```python
from build123d import *

# Parameters (mm, degrees)
F1_DEPTH  = 19.05
F2_R      = 5.08
F3_W      = 76.2
F3_H      = 101.6
F4_DEPTH  = 9.525
F6_DEPTH  = 12.7
F8_DEPTH  = 25.4
F10_DEPTH = 3.175
F12_DEPTH = 6.35
F14_DEPTH = 6.35


with BuildPart() as f1:
    # F0 (on Top) → F1 (new body)
    with BuildSketch(Plane.XY):
        with BuildLine():
            ThreePointArc((41.275, 47.625), (39.4151280605, 52.1151280605), (34.925, 53.975))
            Line((34.925, 53.975), (-34.925, 53.975))
            ThreePointArc((-34.925, 53.975), (-39.4151280605, 52.1151280605), (-41.275, 47.625))
            Line((-41.275, 47.625), (-41.275, -47.625))
            ThreePointArc((-41.275, -47.625), (-39.4151280605, -52.1151280605), (-34.925, -53.975))
            Line((-34.925, -53.975), (34.925, -53.975))
            ThreePointArc((34.925, -53.975), (39.4151280605, -52.1151280605), (41.275, -47.625))
            Line((41.275, -47.625), (41.275, 47.625))
        make_face()
    extrude(amount=F1_DEPTH)

    # F2
    f2_edges = [f1.edges().sort_by_distance(p)[0] for p in [
        (0, -53.975, 0),
    ]]
    fillet(f2_edges, radius=F2_R)

    # F3 (on face) → F4 (cut)
    with BuildSketch(Plane.XY.offset(19.05)):
        Rectangle(F3_W, F3_H)
    extrude(amount=-F4_DEPTH, mode=Mode.SUBTRACT)

    # F5 (on face) → F6 (cut)
    with BuildSketch(Plane.XY.offset(19.05)):
        with BuildLine():
            ThreePointArc((-34.925, 53.975), (-38.1, 53.124261314), (-40.424261314, 50.8))
            Line((-40.424261314, 50.8), (-38.1, 50.8))
            Line((-38.1, 50.8), (38.1, 50.8))
            Line((38.1, 50.8), (40.424261314, 50.8))
            ThreePointArc((40.424261314, 50.8), (38.1, 53.124261314), (34.925, 53.975))
            Line((34.925, 53.975), (-34.925, 53.975))
        make_face()
    extrude(amount=-F6_DEPTH, mode=Mode.SUBTRACT)

    # F7 (on face) → F8 (cut)
    with BuildSketch(Plane(origin=(38.1, 0, 0), x_dir=(0, -1, 0), z_dir=(-1, 0, 0))):
        Polygon((34.925, 15.875), (34.925, 19.05), (-50.8, 19.05), (-50.8, 9.525), (50.8, 9.525), (50.8, 15.875), align=None)
    extrude(amount=-F8_DEPTH, mode=Mode.SUBTRACT)

    # F9 (on face) → F10 (cut)
    with BuildSketch(Plane.YZ.offset(-38.1)):
        Polygon((50.8, 19.05), (-34.925, 19.05), (-34.925, 15.875), (-50.8, 15.875), (-50.8, 9.525), (50.8, 9.525), align=None)
    extrude(amount=-F10_DEPTH, mode=Mode.SUBTRACT)

    # F11 (on face) → F12 (join)
    with BuildSketch(Plane(origin=(0, 0, 15.875), x_dir=(1, 0, 0), z_dir=(0, 0, -1))):
        with BuildLine():
            Line((38.1, 47.625), (41.275, 47.625))
            ThreePointArc((41.275, 47.625), (41.0586289969, 49.2685009364), (40.424261314, 50.8))
            Line((40.424261314, 50.8), (38.1, 50.8))
            Line((38.1, 50.8), (38.1, 47.625))
        make_face()
    extrude(amount=F12_DEPTH)

    # F13 (on face) → F14 (join)
    with BuildSketch(Plane(origin=(0, 0, 15.875), x_dir=(1, 0, 0), z_dir=(0, 0, -1))):
        with BuildLine():
            ThreePointArc((-40.424261314, 50.8), (-41.0586289969, 49.2685009364), (-41.275, 47.625))
            Line((-41.275, 47.625), (-38.1, 47.625))
            Line((-38.1, 47.625), (-38.1, 50.8))
            Line((-38.1, 50.8), (-40.424261314, 50.8))
        make_face()
    extrude(amount=F14_DEPTH)


solid = f1.part
```
The listing builds one solid part. Answer for the finished solid, in the listing's coordinates (mm). A direction names the side the tool comes from. Give positions to 0.01 mm unless a question says otherwise; leave off trailing zeros. Order: outer loops, then holes, each group sorted by start corner. A loop starts at its lowest first (then second) coordinate and runs counter-clockwise, first axis right, second up.
Item 1: For a pull along Z with two mould halves and no side action, classify faces 4 (the face through (-41.275, 1, 7)), 5 (the face through (39.8, 0.7, 1.5)), 6 (the face through (40, -47.625, 13)) as pulls with the +Z half, pulls with the -Z half, needs draft (parallel to the pull), parting line crosses it, or undercut.
From the geometry:
face 4: needs draft
face 5: pulls with the -Z half
face 6: undercut
Item 2: Find the intervals of material crossed by probe 1 along Y at (x, z) = (-15, 18) (3 decimals); probe 2 along Z at (x, y) = (-21, -43.5) (3 decimals); probe 3 along Y at (x, z) = (28.5, 9) (3 decimals), in increasing order.
From the geometry:
probe 1: y = -53.975 to -50.8
probe 2: z = 0 to 9.525
probe 3: y = -53.975 to 50.8
Item 3: The part is cut by section D-D, the plane y = 43.5. Give the vertices of the cut face in (x, z) (3 decimals).
From the geometry:
outline: (-41.275, 5.08) arc R5.08 ccw to (-36.195, 0) - (36.195, 0) arc R5.08 ccw to (41.275, 5.08) - (41.275, 9.525) - (-41.275, 9.525) - close
Item 4: The part is cut by section A-A, the plane y = -42.5. Give the vertices of the cut face in (x, z) (3 decimals).
From the geometry:
outline: (-41.275, 5.08) arc R5.08 ccw to (-36.195, 0) - (36.195, 0) arc R5.08 ccw to (41.275, 5.08) - (41.275, 9.525) - (-41.275, 9.525) - close; (-41.275, 15.875) - (-38.1, 15.875) - (-38.1, 19.05) - (-41.275, 19.05) - close; (38.1, 15.875) - (41.275, 15.875) - (41.275, 19.05) - (38.1, 19.05) - close
Item 5: Which of the six approach directions +Z, -Z, +X, -X, +Y, -Y give full straight-line access (tool end or side, diameter ignored) to faces 1 (the face through (-1, -50.8, 14)), 2 (the face through (-40, -41, 15.875)), 3 (the face through (-1, 52, 6.35))?
From the geometry:
face 1: +Z, +Y
face 2: +X, -X, +Y
face 3: +Z, +X, -X, +Y
Item 6: The part is cut by section B-B, the plane z = 13.75. Give the vertices of the cut face in (x, y) (3 decimals).
From the geometry:
outline: (-41.275, -47.625) arc R6.35 ccw to (-34.925, -53.975) - (34.925, -53.975) arc R6.35 ccw to (41.275, -47.625) - (38.1, -47.625) - (38.1, -50.8) - (-38.1, -50.8) - (-38.1, -47.625) - close
Item 7: The part is cut by section C-C, the plane x = -29.5. Give the vertices of the cut face in (y, z) (3 decimals), and give its area (3 significant figures).
From the geometry:
outline: (-53.975, 5.08) arc R5.08 ccw to (-48.895, 0) - (48.895, 0) arc R5.08 ccw to (53.975, 5.08) - (53.975, 6.35) - (50.8, 6.35) - (50.8, 9.525) - (-50.8, 9.525) - (-50.8, 19.05) - (-53.975, 19.05) - close
area: 1,040 mm2
Item 8: Given pin 1 Ø25 at (x, y) = (-17, 19) entering from +Z (3 decimals); pin 2 Ø2.5 at (x, y) = (-40, -40.5) entering from -Z; pin 3 Ø3.5 at (x, z) = (40, 17) entering from +Y (3 decimals), each flat-ended and moving along its own axis, determine where each tip first touches the part or whether it passes through.
From the geometry:
pin 1: stops at z = 9.525
pin 2: stops at z = 0.69
pin 3: stops at y = -34.925
